from build123d import *

# Parameters (mm, degrees)
SKETCH1_R           = 11.1125
BOSS_EXTRUDE1_DEPTH = 5.9944
SKETCH2_W           = 38.1
SKETCH2_H           = 1.5875
CUT_EXTRUDE1_DEPTH  = 6.9944


with BuildPart() as part:
    # Sketch1 → Boss-Extrude1 (new body)
    with BuildSketch(Plane.XY):
        Polygon((19.05, 19.05), (-19.05, 19.05), (-19.05, 12.7), (-25.0444, 12.7), (-25.0444, 0), (-19.05, 0), (-19.05, -12.7), (-25.0444, -12.7), (-25.0444, -25.4), (-19.05, -25.4), (-19.05, -31.75), (19.05, -31.75), (19.05, -25.4), (25.0444, -25.4), (25.0444, -12.7), (19.05, -12.7), (19.05, 0), (25.0444, 0), (25.0444, 12.7), (19.05, 12.7), align=None)
        Circle(SKETCH1_R, mode=Mode.SUBTRACT)
    extrude(amount=BOSS_EXTRUDE1_DEPTH)

    # Sketch2 → Cut-Extrude1 (cut, through all)
    with BuildSketch(Plane.XY.offset(5.9944)):
        with Locations((0, -30.95625)):
            Rectangle(SKETCH2_W, SKETCH2_H)
        with Locations((0, 18.25625)):
            Rectangle(SKETCH2_W, SKETCH2_H)
    extrude(amount=-CUT_EXTRUDE1_DEPTH, mode=Mode.SUBTRACT)


solid = part.part
Verification items for the finished model (mm, model axes). A direction names the side the tool comes from. Give positions to 0.01 mm unless a question says otherwise; leave off trailing zeros. Loops run counter-clockwise (first coordinate to the right, second up) from the corner with the lowest first, then second, coordinate; pieces in that order, holes last.
1) Depth check by flat-ended pin: pin 1 Ø1.8 at (x, z) = (23.5, 3.5) entering from +Y; pin 2 Ø1.4 at (y, z) = (-27, 2.5) entering from +X. Enter the tip coordinate at first touch or a pass-through.
2) Sectioned sample at D-D, the plane y = 13.5. Enter the section's corners in (x, z), then the cut area to 3 significant figures.
3) Sectioned sample at A-A, the plane x = 0. Enter the section's corners in (y, z).
4) Sectioned sample at C-C, the plane y = -8.5. Enter the section's corners in (x, z), then the cut area to 3 significant figures.
5) Set-up check for faces 1 (the flat face through (-22, -25.4, 3)), 2 (the flat face through (22, -12.7, 3)), 3 (the flat face through (19.05, -28, 3)): record each of +Z, -Z, +X, -X, +Y, -Y from which the full face is reachable in a straight line by a thin tool's end or side.
6) Thickness scan on line 1 along X through (y, z) = (-0.5, 2.45); line 2 along Y through (x, z) = (0, 4.2); line 3 along Y through (x, z) = (-21.5, 0.55). Record the ranges inside material, lowest first.
7) Draft check along Y on faces 4 (the flat face through (22, 12.7, 3)), 5 (the flat face through (0, -30.162, 3)), 6 (the flat face through (-22, 0, 3)). Enter one of: pulls with the +Y half, pulls with the -Y half, needs draft (parallel to the pull), parting line crosses it, or undercut.
Answers:
1. pin 1: stops at y = 12.7
1. pin 2: stops at x = 19.05
2. outline: (-19.05, 0) - (19.05, 0) - (19.05, 5.99) - (-19.05, 5.99) - close
2. area: 228 mm2
3. outline: (-30.16, 0) - (-11.11, 0) - (-11.11, 5.99) - (-30.16, 5.99) - close; (11.11, 0) - (17.46, 0) - (17.46, 5.99) - (11.11, 5.99) - close
4. outline: (-19.05, 0) - (-7.16, 0) - (-7.16, 5.99) - (-19.05, 5.99) - close; (7.16, 0) - (19.05, 0) - (19.05, 5.99) - (7.16, 5.99) - close
4. area: 143 mm2
5. face 1: +Z, -Z, -X, -Y
5. face 2: +Z, -Z, +X
5. face 3: +Z, -Z, +X, -Y
6. line 1: x = -19.05 to -11.1, 11.1 to 19.05
6. line 2: y = -30.16 to -11.11, 11.11 to 17.46
6. line 3: y = -25.4 to -12.7, 0 to 12.7
7. face 4: pulls with the +Y half
7. face 5: pulls with the -Y half
7. face 6: undercut
